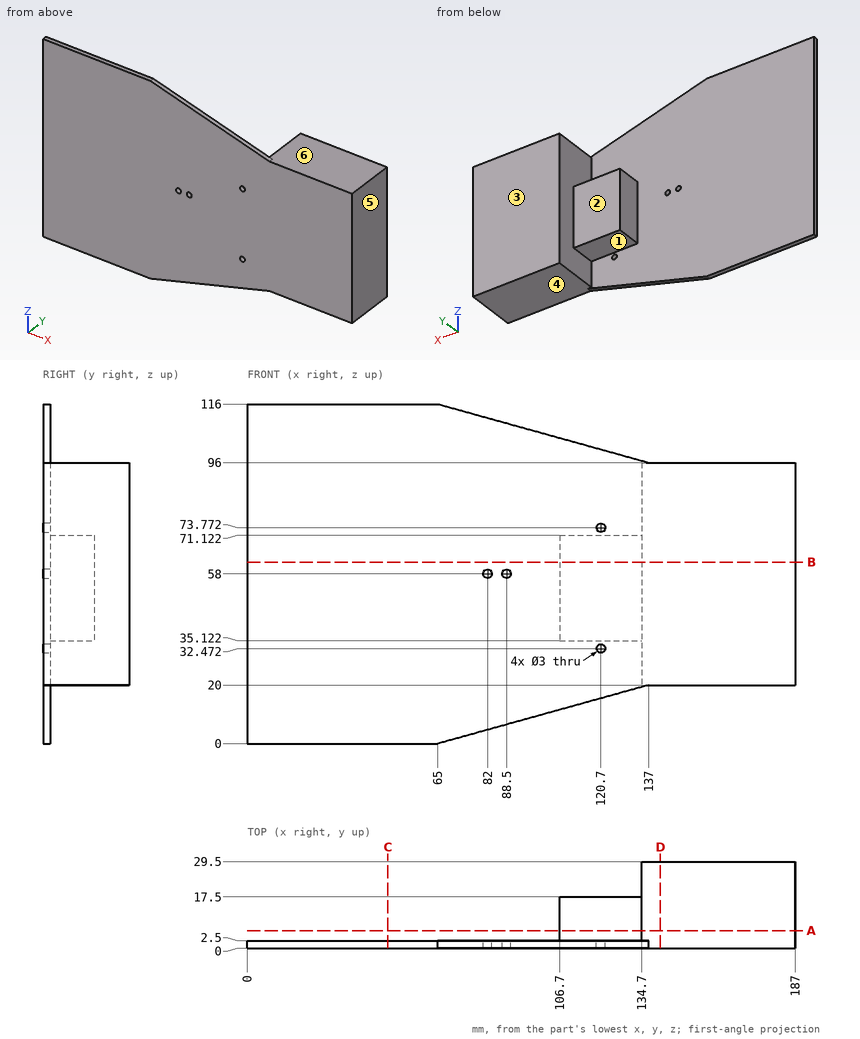
Here's the drawing with two shaded views (mm, measured from the low corner). I have some questions. A direction names the side the tool comes from. Coordinates: 2 decimals unless noted, no trailing zeros. Loops run counter-clockwise (first coordinate to the right, second up) from the corner with the lowest first, then second, coordinate; pieces in that order, holes last. Notation, with made-up numbers: M 43,-39 L 89,-39 A18 ccw 89,-4 Z; hole C 15.5,29.5 d8. An arc over 180 degrees is marked long. Return JSON: item names as keys, results as strings. Group by question number.
Item 1: Imagine slicing it at A-A (y = 6). Please give me the cut outline in (x, z), and give its area (3 significant figures).
Item 2: Thinking about a two-plate mould opening in Z: for the marked faces 4, 5 and 6, which applies, released by +Z, released by -Z, zero draft, split by the parting line, or undercut?
Item 3: Imagine slicing it at B-B (z = 62). Please give me the cut outline in (x, y).
Item 4: Imagine slicing it at C-C (x = 48). Please give me the cut outline in (y, z), and give its area (3 significant figures).
Item 5: I'm going to push flat-ended pins straight in: pin 1 Ø9 at (x, y) = (159, 11.5) entering from -Z; pin 2 Ø1.8 at (x, z) = (120.7, 32.47) entering from -Y; pin 3 Ø1.5 at (y, z) = (5.5, 81) entering from -X; pin 4 Ø14 at (x, z) = (127.5, 61.5) entering from +Y. Where does each tip first touch, or does it pass through?
Item 6: Imagine slicing it at D-D (x = 141). Please give me the cut outline in (y, z).
Item 7: If I drill on L1, parallel to X at y = 1.95, z = 58; L2, parallel to Z at x = 120.7, y = 1.4; L3, parallel to Y at x = 126.5, z = 75.5, over which ranges is the centre line in solid material (lowest first)? Write a range as from..to.
Item 8: On a 3-axis mill with a long thin cutter (end or side, diameter ignored), from which of +Z, -Z, +X, -X, +Y, -Y can I reach the whole of each face in a straight line? I mean the marked faces 1, 2 and 3. Say none if no direction works.
Verdict:
{
 "1": {"outline": "M 106.7,35.12 L 134.7,35.12 L 134.7,20 L 187,20 L 187,96 L 134.7,96 L 134.7,71.12 L 106.7,71.12 Z", "area": "4,980 mm^2"},
 "2": {"face 4": "released by -Z", "face 5": "zero draft", "face 6": "released by +Z"},
 "3": {"outline": "M 0,0 L 187,0 L 187,29.5 L 134.7,29.5 L 134.7,17.5 L 106.7,17.5 L 106.7,2.5 L 0,2.5 Z"},
 "4": {"outline": "M 0,0 L 2.5,0 L 2.5,116 L 0,116 Z", "area": "290 mm^2"},
 "5": {"pin 1": "stops at z = 20", "pin 2": "passes through", "pin 3": "stops at x = 134.7", "pin 4": "stops at y = 17.5"},
 "6": {"outline": "M 0,20 L 29.5,20 L 29.5,96 L 0,96 Z"},
 "7": {"L1": "x = 0..80.5, 83.5..87, 90..187", "L2": "z = 15.47..30.97, 33.97..72.27, 75.27..100.53", "L3": "y = 0..2.5"},
 "8": {"face 1": "-Z, -X, +Y", "face 2": "+Z, -Z, -X, +Y", "face 3": "+Z, -Z, +X, -X, +Y"}
}
